```python
from build123d import *

# Parameters (mm, degrees)
SKETCH1_R               = 1.5
BOSS_EXTRUDE1_DEPTH     = 6
CUT_EXTRUDE1_DEPTH      = 21.506096654
CUT_EXTRUDE1_DEPTH_BACK = 21.506096654
SKETCH2_W               = 12
SKETCH2_H               = 6
SKETCH3_R               = 2
CUT_EXTRUDE2_DEPTH      = 10


with BuildPart() as part:
    # Sketch1 → Boss-Extrude1 (new, symmetric)
    with BuildSketch(Plane.XY):
        with BuildLine():
            Line((-18.5, 6.5), (0, 6.5))
            ThreePointArc((0, 6.5), (6.5, 0), (0, -6.5))
            Line((0, -6.5), (-18.5, -6.5))
            Line((-18.5, -6.5), (-18.5, 6.5))
        make_face()
        with Locations((0, 3.5)):
            Circle(SKETCH1_R, mode=Mode.SUBTRACT)
        with Locations(Location((0, -3.5, 0), (0, 0, 180))):
            Circle(SKETCH1_R, mode=Mode.SUBTRACT)
    extrude(amount=BOSS_EXTRUDE1_DEPTH, both=True)

    # Sketch2 → Cut-Extrude1 (cut, two sides: drawn at the far end of the back side and taken through both)
    with BuildSketch(Plane(origin=(0, 0, 0), x_dir=(1, 0, 0), z_dir=(0, 1, 0)).offset(-CUT_EXTRUDE1_DEPTH_BACK)):
        with Locations((0.5, 0)):
            Rectangle(SKETCH2_W, SKETCH2_H)
    extrude(amount=CUT_EXTRUDE1_DEPTH + CUT_EXTRUDE1_DEPTH_BACK, mode=Mode.SUBTRACT)

    # Sketch3 → Cut-Extrude2 (cut)
    with BuildSketch(Plane.ZY.offset(18.5)):
        Circle(SKETCH3_R)
    extrude(amount=-CUT_EXTRUDE2_DEPTH, mode=Mode.SUBTRACT)


solid = part.part
```
The model under review builds one solid part; all positions refer to its coordinate system, in mm. A direction names the side the tool comes from. Round coordinates to 2 decimals unless told otherwise and drop trailing zeros. Write each loop counter-clockwise with the first axis right and the second up, starting at its lowest first coordinate (ties: lowest second). Pieces come first, ordered by that corner, then holes. Notation, with made-up numbers: (46, -27.75) - (69, -27.75) arc R27 ccw to (69, 5.25) - close; hole circle Ø11 at (85.25, 32). An arc over 180 degrees is marked (long way). Use one line per item in the form item = value.
Q1. For line 1 (Z direction, x = -3.75, y = 4); line 2 (Y direction, x = -11, z = 0); line 3 (Y direction, x = 1.25, z = 4.25), list the stretches that pass through material, from the lowest coordinate up. Write a range as [from, to].
Answer key:
line_1 = [-6, -3], [3, 6]
line_2 = [-6.5, -2], [2, 6.5]
line_3 = [-6.38, -4.33], [-2.67, 2.67], [4.33, 6.38]
Q2. Consider section C-C (z = 4.5). State the section outline as (x, y) points, and give its area (3 significant figures).
Answer key:
outline = (-18.5, -6.5) - (0, -6.5) arc R6.5 ccw to (0, 6.5) - (-18.5, 6.5) - close; hole circle Ø3 at (0, -3.5); hole circle Ø3 at (0, 3.5)
area = 293 mm2
Q3. Consider section B-B (y = -2.25). State the section outline as (x, z) points, and give its area (3 significant figures).
Answer key:
outline = (-18.5, -6) - (-0.83, -6) - (-0.83, -3) - (-5.5, -3) - (-5.5, 3) - (-0.83, 3) - (-0.83, 6) - (-18.5, 6) - close; (0.83, -6) - (6.1, -6) - (6.1, -3) - (0.83, -3) - close; (0.83, 3) - (6.1, 3) - (6.1, 6) - (0.83, 6) - close
area = 216 mm2
Q4. Insertion check: pin 1 Ø1.8 at (y, z) = (0.5, 1) entering from +X; pin 2 Ø2.5 at (x, y) = (0, 3.5) entering from +Z; pin 3 Ø2 at (y, z) = (0, 0.5) entering from -X; pin 4 Ø3 at (y, z) = (-4.5, -4.5) entering from +X. Each pin has a flat end and moves straight along its axis. Give the tip position at first contact, or say it passes through.
Answer key:
pin_1 = -5.5
pin_2 = through
pin_3 = -8.5
pin_4 = 5.77
Q5. Tool access review of faces 1 (the flat face through (0, 0, -3)), 2 (the cylindrical face through (-14, -2, 0)), 3 (the cylindrical face through (6.5, 0.1, 4.5)): name each direction out of +Z, -Z, +X, -X, +Y, -Y from which nothing blocks a thin tool from reaching the whole face with its end or side.
Answer key:
face_1 = +X, +Y, -Y
face_2 = -X
face_3 = +Z, -Z, +X
Q6. Consider section D-D (x = -1). State the section outline as (y, z) points, and give its area (3 significant figures).
Answer key:
outline = (-6.5, -6) - (-4.62, -6) - (-4.62, -3) - (-6.5, -3) - close; (-6.5, 3) - (-4.62, 3) - (-4.62, 6) - (-6.5, 6) - close; (-2.38, -6) - (2.38, -6) - (2.38, -3) - (-2.38, -3) - close; (-2.38, 3) - (2.38, 3) - (2.38, 6) - (-2.38, 6) - close; (4.62, -6) - (6.5, -6) - (6.5, -3) - (4.62, -3) - close; (4.62, 3) - (6.5, 3) - (6.5, 6) - (4.62, 6) - close
area = 51.2 mm2
Q7. Draft analysis for pull direction Y (two halves, no side actions). For faces 4 (the flat face through (-6, 0, -6)), 5 (the cylindrical face through (6.5, 0.1, -4.5)), 6 (the cylindrical face through (-1.5, 3.57, 4.48)), state which applies: +Y half, -Y half, draft (parallel to the pull), parting line (faces both ways), or undercut.
Answer key:
face_4 = draft
face_5 = parting line
face_6 = undercut
Q8. Consider section A-A (x = -5). State the section outline as (y, z) points, and give its area (3 significant figures).
Answer key:
outline = (-6.5, -6) - (6.5, -6) - (6.5, -3) - (-6.5, -3) - close; (-6.5, 3) - (6.5, 3) - (6.5, 6) - (-6.5, 6) - close
area = 78.0 mm2
